Autodesk Inventor part; units mm, degrees
ref_plane "YZ Plane" through (0, 0, 0) normal (1, 0, 0) x (0, 1, 0)
ref_plane "XZ Plane" through (0, 0, 0) normal (0, 1, 0) x (-1, 0, 0)
ref_plane "XY Plane" through (0, 0, 0) normal (0, 0, 1) x (1, 0, 0)
sketch "Sketch1" plane through (0, 0, 0) normal (0, 0, 1) x (1, 0, 0)
  line L0 (0, -0.996467) -> (0, 5.9788) construction
  line L1 (-0.996467, 0) -> (5.9788, 0) construction
  line L2 (4.1275, 0) -> (4.1275, 4.7625)
  line L3 (4.1275, 4.7625) -> (0, 4.7625)
  line L4 (0, 4.7625) -> (0, 4.1275)
  arc A0 (4.1275, 0) -> (0, 4.1275) centre (0, 0) ccw
  point P0 (0, 0)
  dimension "d0" = 4.7625
  dimension "d1" = 4.1275
  dimension "d2" = 0.635
  dimension "d3" = 4.1275
sketch "Sketch1 outline for Revolution1" plane through (0, 0, 0) normal (0, 0, 1) x (1, 0, 0)
  arc A0 (0, 4.1275) -> (4.1275, 0) centre (0, 0) cw
  line L0 (0, 4.7625) -> (0, 4.1275)
  line L1 (4.1275, 4.7625) -> (0, 4.7625)
  line L2 (4.1275, 0) -> (4.1275, 4.7625)
revolve "Revolution1" add sketch "Sketch1 outline for Revolution1" angle 360 about axis through (0, -10, 0) along (0, 1, 0)
fillet "Fillet1" radius 0.381 2 edges at (-4.1275, 4.7625, 0) (-4.1275, 0, 0)
sketch "Sketch2" plane through (0, 4.7625, 0) normal (0, 1, 0) x (1, 0, 0)
  circle A0 centre (0, 0) radius 2.06375
  dimension "d6" = 4.1275
sketch "Sketch2 outline for Extrusion1" plane through (0, 4.7625, 0) normal (0, 1, 0) x (1, 0, 0)
  circle A0 centre (0, 0) radius 2.06375
extrude "Extrusion1" cut sketch "Sketch2 outline for Extrusion1" along normal through all both and the other way through all
properties part number "Pillow Ball Bushing"
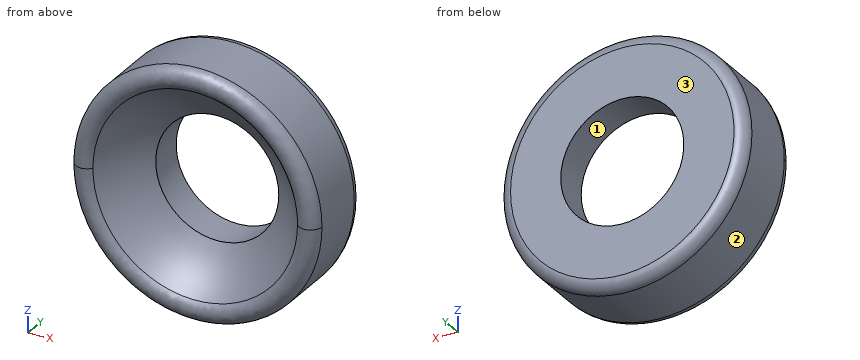
Design review of the part built by this model. Coordinates are the model's own, in mm. Face numbers are marked on the shaded views. Coordinates: 2 decimals unless noted, no trailing zeros. Order: outer loops, then holes, each group sorted by start corner. A loop starts at its lowest first (then second) coordinate and runs counter-clockwise, first axis right, second up. Notation, with made-up numbers: M -34,67.5 L -8,67.5 A23 cw -8,75.5 Z; hole C 21,86 d2. An arc over 180 degrees is marked long. Answer as a JSON object with one key per item and string values. Group by question number.
1) Wall thickness on L1, parallel to X at y = 3.95, z = 0; L2, parallel to X at y = 2.65, z = -1.75: over which ranges is each line inside the solid? List them lowest first.
2) Add section B-B, the plane y = 3.15. Write out the cut boundary in (x, z) (1 decimal), then the cut area to 3 significant figures.
3) Add section A-A, the plane y = 3.85. Write out the cut boundary in (x, z) (1 decimal).
4) For pin 1 (1.5 mm diameter, centred on x = -1, y = 2.5, fed in from -Z); pin 2 (3.5 mm diameter, centred on x = 0, z = 0, fed in from -Y), all flat-tipped, find the tip position at first contact; note any pin that passes through.
5) Mouldability with a two-part tool opening along X and no side actions: class the marked faces 1, 2 and 3 as pulls with the +X half, pulls with the -X half, needs draft (parallel to the pull), parting line crosses it, or undercut.
Computed values:
{
 "1": {"L1": "x = -4.13 to -2.06, 2.06 to 4.13", "L2": "x = -3.74 to -2.64, 2.64 to 3.74"},
 "2": {"outline": "C 0,0 d8.3; hole C 0,0 d5.3", "area": "31.2 mm^2"},
 "3": {"outline": "C 0,0 d8.3; hole C 0,0 d4.1"},
 "4": {"pin 1": "stops at z = -4.12", "pin 2": "passes through"},
 "5": {"face 1": "undercut", "face 2": "parting line crosses it", "face 3": "needs draft"}
}
